Part model, mm, in its own coordinate system. Face numbers are marked on the shaded views. A direction names the side the tool comes from. Round coordinates to 2 decimals unless told otherwise and drop trailing zeros. Order: outer loops, then holes, each group sorted by start corner. A loop starts at its lowest first (then second) coordinate and runs counter-clockwise, first axis right, second up. Notation, with made-up numbers: (5.25, 22.25) - (36.25, 22.25) arc R11 cw to (36.25, 31.25) - close; hole circle Ø3 at (76, -16.75). An arc over 180 degrees is marked (long way). Return JSON: item names as keys, results as strings. Group by question number.
Item 1: Probe probe 1 along Y at (x, z) = (27.75, 0.95) (3 decimals); probe 2 along X at (y, z) = (-8, 8); probe 3 along Z at (x, y) = (-17, -6.5). List the from-to ranges inside material, lowest first.
Item 2: Saw through at A-A on x = -27.75. List the corners of the cut face in (y, z) (3 decimals).
Item 3: Two-plate mould, pull along X, no slides. Class the marked faces 3, 4 and 5: released by +X, released by -X, zero draft, split by the parting line, or undercut.
Item 4: Saw through at D-D on z = 8.5. List the corners of the cut face in (x, y), and give its area (3 significant figures).
Item 5: Drop flat-ended pins along their axis: pin 1 (4 mm diameter, centred on x = -0.5, z = 5, fed in from +Y) (3 decimals); pin 2 (0.8 mm diameter, centred on x = 51.5, z = 6.5, fed in from -Y); pin 3 (3.5 mm diameter, centred on x = -19, y = -15, fed in from +Z); pin 4 (1.2 mm diameter, centred on x = 51, z = 7, fed in from +Y). Give the stop position or say it passes through.
Item 6: Tool access for the marked faces 1 and 2: list every direction of +Z, -Z, +X, -X, +Y, -Y with a clear straight run to the whole face (end or side of a thin tool).
Item 7: Saw through at B-B on y = -4. List the corners of the cut face in (x, z), and give its area (3 significant figures).
Item 8: Saw through at C-C on y = 0. List the corners of the cut face in (x, z).
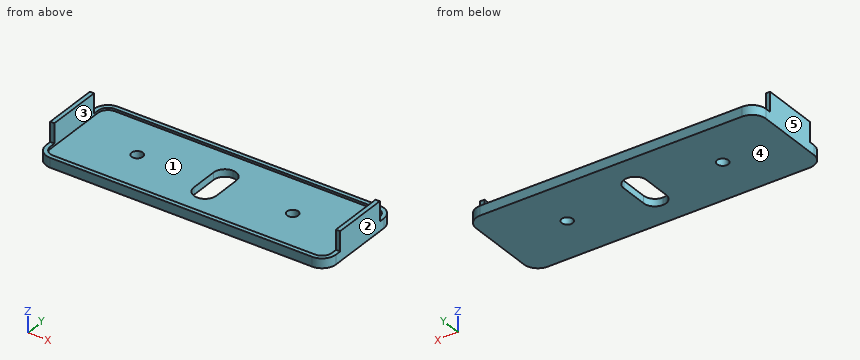
```python
from build123d import *

# Parameters (mm, degrees)
SKETCH1_R           = 2
BOSS_EXTRUDE1_DEPTH = 3.4
CUT_EXTRUDE1_START  = -0.8
SKETCH2_R           = 2
CUT_EXTRUDE1_DEPTH  = 0.8
SKETCH3_W           = 1.5
SKETCH3_H           = 20
BOSS_EXTRUDE2_DEPTH = 7


with BuildPart() as part:
    # Sketch1 → Boss-Extrude1 (new body)
    with BuildSketch(Plane.XY):
        with BuildLine():
            Line((-46.75, 17.075), (46.75, 17.075))
            ThreePointArc((46.75, 17.075), (50.285533906, 15.610533906), (51.75, 12.075))
            Line((51.75, 12.075), (51.75, -12.075))
            ThreePointArc((51.75, -12.075), (50.285533906, -15.610533906), (46.75, -17.075))
            Line((46.75, -17.075), (-46.75, -17.075))
            ThreePointArc((-46.75, -17.075), (-50.285533906, -15.610533906), (-51.75, -12.075))
            Line((-51.75, -12.075), (-51.75, 12.075))
            ThreePointArc((-51.75, 12.075), (-50.285533906, 15.610533906), (-46.75, 17.075))
        make_face()
        with Locations((-27.75, 0)):
            Circle(SKETCH1_R, mode=Mode.SUBTRACT)
        with Locations((27.75, 0)):
            Circle(SKETCH1_R, mode=Mode.SUBTRACT)
        with BuildLine():
            Line((-0.01, 9), (0.01, 9))
            ThreePointArc((0.01, 9), (2.831356057, 7.831356057), (4, 5.01))
            Line((4, 5.01), (4, -5.01))
            ThreePointArc((4, -5.01), (2.831356057, -7.831356057), (0.01, -9))
            Line((0.01, -9), (-0.01, -9))
            ThreePointArc((-0.01, -9), (-2.831356057, -7.831356057), (-4, -5.01))
            Line((-4, -5.01), (-4, 5.01))
            ThreePointArc((-4, 5.01), (-2.831356057, 7.831356057), (-0.01, 9))
        make_face(mode=Mode.SUBTRACT)
    extrude(amount=BOSS_EXTRUDE1_DEPTH)

    # Sketch2 → Cut-Extrude1 (cut)
    with BuildSketch(Plane.XY.offset(3.4).offset(CUT_EXTRUDE1_START)):
        with BuildLine():
            Line((50.25, -12.075), (50.25, 12.075))
            ThreePointArc((50.25, 12.075), (49.224873734, 14.549873734), (46.75, 15.575))
            Line((46.75, 15.575), (-46.75, 15.575))
            ThreePointArc((-46.75, 15.575), (-49.224873734, 14.549873734), (-50.25, 12.075))
            Line((-50.25, 12.075), (-50.25, -12.075))
            ThreePointArc((-50.25, -12.075), (-49.224873734, -14.549873734), (-46.75, -15.575))
            Line((-46.75, -15.575), (46.75, -15.575))
            ThreePointArc((46.75, -15.575), (49.224873734, -14.549873734), (50.25, -12.075))
        make_face()
        with Locations((-27.75, 0)):
            Circle(SKETCH2_R, mode=Mode.SUBTRACT)
        with Locations((27.75, 0)):
            Circle(SKETCH2_R, mode=Mode.SUBTRACT)
        with BuildLine():
            ThreePointArc((0.01, 9), (2.831356057, 7.831356057), (4, 5.01))
            Line((4, 5.01), (4, -5.01))
            ThreePointArc((4, -5.01), (2.831356057, -7.831356057), (0.01, -9))
            Line((0.01, -9), (-0.01, -9))
            ThreePointArc((-0.01, -9), (-2.831356057, -7.831356057), (-4, -5.01))
            Line((-4, -5.01), (-4, 5.01))
            ThreePointArc((-4, 5.01), (-2.831356057, 7.831356057), (-0.01, 9))
            Line((-0.01, 9), (0.01, 9))
        make_face(mode=Mode.SUBTRACT)
    extrude(amount=CUT_EXTRUDE1_DEPTH, mode=Mode.SUBTRACT)

    # Sketch3 → Boss-Extrude2 (add)
    with BuildSketch(Plane.XY.offset(3.4)):
        with Locations((-51, 0)):
            Rectangle(SKETCH3_W, SKETCH3_H)
    boss_extrude2 = extrude(amount=BOSS_EXTRUDE2_DEPTH)

    # Mirror1: Boss-Extrude2 across plane
    add(boss_extrude2.mirror(Plane(origin=(0, 0, 0), x_dir=(0, 0, 1), z_dir=(1, 0, 0))))


solid = part.part
```
Filled in:
{
 "1": {"probe 1": "y = -17.075 to -2, 2 to 17.075", "probe 2": "x = -51.75 to -50.25, 50.25 to 51.75", "probe 3": "z = 0 to 2.6"},
 "2": {"outline": "(-17.075, 0) - (-2, 0) - (-2, 2.6) - (-15.575, 2.6) - (-15.575, 3.4) - (-17.075, 3.4) - close; (2, 0) - (17.075, 0) - (17.075, 3.4) - (15.575, 3.4) - (15.575, 2.6) - (2, 2.6) - close"},
 "3": {"face 3": "undercut", "face 4": "zero draft", "face 5": "released by -X"},
 "4": {"outline": "(-51.75, -10) - (-50.25, -10) - (-50.25, 10) - (-51.75, 10) - close; (50.25, -10) - (51.75, -10) - (51.75, 10) - (50.25, 10) - close", "area": "60.0 mm^2"},
 "5": {"pin 1": "stops at y = 17.075", "pin 2": "stops at y = -10", "pin 3": "stops at z = 3.4", "pin 4": "stops at y = 10"},
 "6": {"face 1": "+Z", "face 2": "+Z, -Z, +X, +Y, -Y"},
 "7": {"outline": "(-51.75, 0) - (-4, 0) - (-4, 2.6) - (-50.25, 2.6) - (-50.25, 10.4) - (-51.75, 10.4) - close; (4, 0) - (51.75, 0) - (51.75, 10.4) - (50.25, 10.4) - (50.25, 2.6) - (4, 2.6) - close", "area": "272 mm^2"},
 "8": {"outline": "(-51.75, 0) - (-29.75, 0) - (-29.75, 2.6) - (-50.25, 2.6) - (-50.25, 10.4) - (-51.75, 10.4) - close; (-25.75, 0) - (-4, 0) - (-4, 2.6) - (-25.75, 2.6) - close; (4, 0) - (25.75, 0) - (25.75, 2.6) - (4, 2.6) - close; (29.75, 0) - (51.75, 0) - (51.75, 10.4) - (50.25, 10.4) - (50.25, 2.6) - (29.75, 2.6) - close"}
}
